Check sheet for the modelled part. Datum: model origin and axes. Units: mm. Face numbers are marked on the shaded views. A direction names the side the tool comes from. Round coordinates to 2 decimals unless told otherwise and drop trailing zeros. Write each loop counter-clockwise with the first axis right and the second up, starting at its lowest first coordinate (ties: lowest second). Pieces come first, ordered by that corner, then holes. Notation, with made-up numbers: M 60,10.25 L 72,10.25 A15 cw 72,27.25 Z; hole C 26,24.5 d9. An arc over 180 degrees is marked long. Answer in a Markdown table with one row per item.
```python
from build123d import *

# Parameters (mm, degrees)
SKETCH_W       = 34
SKETCH_H       = 34
PAD_DEPTH      = 400
SKETCH001_R    = 5
HOLE_DEPTH     = 40.001
SKETCH002_R    = 1.75
HOLE001_DEPTH  = 40.001
SKETCH003_R    = 2
HOLE002_DEPTH  = 25
HOLE002_TIPS_R = 2
SKETCH004_W    = 25
SKETCH004_H    = 30
POCKET_DEPTH   = 3


with BuildPart() as part:
    # Sketch → Pad (new body)
    with BuildSketch(Plane.XZ):
        with BuildLine():
            Line((2, 0), (38, 0))
            ThreePointArc((38, 0), (39.414214, 0.585786), (40, 2))
            Line((40, 2), (40, 38))
            ThreePointArc((40, 38), (39.414214, 39.414214), (38, 40))
            Line((38, 40), (2, 40))
            ThreePointArc((2, 40), (0.585786, 39.414214), (0, 38))
            Line((0, 38), (0, 2))
            ThreePointArc((0, 2), (0.585786, 0.585786), (2, 0))
        make_face()
        with Locations((20, 20)):
            Rectangle(SKETCH_W, SKETCH_H, mode=Mode.SUBTRACT)
    extrude(amount=PAD_DEPTH)

    # Sketch001 (on Face5 of Pad) → Hole (cut, through all)
    with BuildSketch(Plane(origin=(0, 0, 40), x_dir=(-1, 0, 0), z_dir=(0, 0, 1))):
        with Locations((-20, 200)):
            Circle(SKETCH001_R)
    extrude(amount=-HOLE_DEPTH, mode=Mode.SUBTRACT)

    # Sketch002 (on Face10 of Hole) → Hole001 (cut, through all)
    with BuildSketch(Plane(origin=(0, 0, 40), x_dir=(-1, 0, 0), z_dir=(0, 0, 1))):
        with Locations((-12.000033, 200.023056)):
            Circle(SKETCH002_R)
        with Locations((-27.999967, 200.023056)):
            Circle(SKETCH002_R)
        with Locations((-20, 192)):
            Circle(SKETCH002_R)
        with Locations((-19.996319, 207.999999)):
            Circle(SKETCH002_R)
    extrude(amount=-HOLE001_DEPTH, mode=Mode.SUBTRACT)

    # Sketch003 (on Face12 of Hole001) → Hole002 (cut)
    with BuildSketch(Plane(origin=(40, 0, 0), x_dir=(0, 0, 1), z_dir=(1, 0, 0))):
        with Locations((28, 175)):
            Circle(SKETCH003_R)
        with Locations((12, 175)):
            Circle(SKETCH003_R)
        with Locations((28, 159.64)):
            Circle(SKETCH003_R)
        with Locations((12, 159.64)):
            Circle(SKETCH003_R)
    extrude(amount=-HOLE002_DEPTH, mode=Mode.SUBTRACT)

    # Hole002 tips → Hole002 tip 1 section 0
    with BuildSketch(Plane(origin=(15, 0, 0), x_dir=(0, 0, 1), z_dir=(1, 0, 0)), mode=Mode.PRIVATE) as hole002_tip_1_s0:
        with Locations((28, 175)):
            Circle(HOLE002_TIPS_R)
    loft([hole002_tip_1_s0.sketch, Vertex(13.798279, -175, 28)], mode=Mode.SUBTRACT)

    # Hole002 tips → Hole002 tip 2 section 0
    with BuildSketch(Plane(origin=(15, 0, 0), x_dir=(0, 0, 1), z_dir=(1, 0, 0)), mode=Mode.PRIVATE) as hole002_tip_2_s0:
        with Locations((12, 175)):
            Circle(HOLE002_TIPS_R)
    loft([hole002_tip_2_s0.sketch, Vertex(13.798279, -175, 12)], mode=Mode.SUBTRACT)

    # Hole002 tips → Hole002 tip 3 section 0
    with BuildSketch(Plane(origin=(15, 0, 0), x_dir=(0, 0, 1), z_dir=(1, 0, 0)), mode=Mode.PRIVATE) as hole002_tip_3_s0:
        with Locations((28, 159.64)):
            Circle(HOLE002_TIPS_R)
    loft([hole002_tip_3_s0.sketch, Vertex(13.798279, -159.64, 28)], mode=Mode.SUBTRACT)

    # Hole002 tips → Hole002 tip 4 section 0
    with BuildSketch(Plane(origin=(15, 0, 0), x_dir=(0, 0, 1), z_dir=(1, 0, 0)), mode=Mode.PRIVATE) as hole002_tip_4_s0:
        with Locations((12, 159.64)):
            Circle(HOLE002_TIPS_R)
    loft([hole002_tip_4_s0.sketch, Vertex(13.798279, -159.64, 12)], mode=Mode.SUBTRACT)

    # Sketch004 (on Face11 of Hole002) → Pocket (cut)
    with BuildSketch(Plane(origin=(0, 0, 0), x_dir=(0, 0, -1), z_dir=(-1, 0, 0))):
        with Locations((-20, 170)):
            Rectangle(SKETCH004_W, SKETCH004_H)
    extrude(amount=-POCKET_DEPTH, mode=Mode.SUBTRACT)


solid = part.part
```
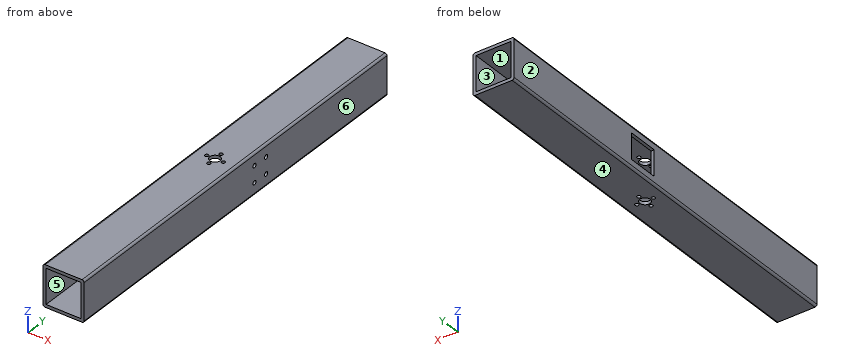
1. Section check A-A, the plane z = 19.5. Record the cut outline in (x, y).
Found:
| item | result |
|---|---|
| outline | M 0,-400 L 3,-400 L 3,-185 L 0,-185 Z; M 0,-155 L 3,-155 L 3,0 L 0,0 Z; M 37,-400 L 40,-400 L 40,0 L 37,0 Z |
2. Go/stop test with flat-tipped pins: pin 1 (0.9 mm diameter, centred on x = 1, y = -165, fed in from -Z); pin 2 (4.5 mm diameter, centred on y = -159.64, z = 28, fed in from -X); pin 3 (3 mm diameter, centred on y = -175, z = 28, fed in from -X). Record where each tip stops, or that it passes through.
Found:
| item | result |
|---|---|
| pin 1 | stops at z = 0.08 |
| pin 2 | stops at x = 37 |
| pin 3 | passes through |
3. Scan lines: L1, parallel to Y at x = 38.3, z = 28; L2, parallel to Z at x = 37.75, y = -159.64; L3, parallel to Y at x = 20, z = 38. Record each from-to range of solid material in increasing order.
Found:
| item | result |
|---|---|
| L1 | y = -400 to -177, -173 to -161.64, -157.64 to 0 |
| L2 | z = 0 to 10, 14 to 26, 30 to 40 |
| L3 | y = -400 to -209.75, -206.25 to -205, -195 to -193.75, -190.25 to 0 |
4. Draft check along X on the marked faces 3, 4, 5 and 6. Enter one of: +X half, -X half, draft (parallel to the pull), parting line (faces both ways), or undercut.
Found:
| item | result |
|---|---|
| face 3 | undercut |
| face 4 | draft |
| face 5 | undercut |
| face 6 | +X half |
5. Section check B-B, the plane y = -223.5. Record the cut outline in (x, z).
Found:
| item | result |
|---|---|
| outline | M 0,2 A2 ccw 2,0 L 38,0 A2 ccw 40,2 L 40,38 A2 ccw 38,40 L 2,40 A2 ccw 0,38 Z; hole M 3,3 L 37,3 L 37,37 L 3,37 Z |
6. Access from +Z, -Z, +X, -X, +Y, -Y to the whole of each face (thin tool, end or side, straight path). Record for the marked faces 1 and 2.
Found:
| item | result |
|---|---|
| face 1 | +Y, -Y |
| face 2 | +Z, -Z, -X, +Y, -Y |
